Design review of the part built by this model. Coordinates are the model's own, in mm. A direction names the side the tool comes from. Coordinates: 2 decimals unless noted, no trailing zeros. Loops run counter-clockwise (first coordinate to the right, second up) from the corner with the lowest first, then second, coordinate; pieces in that order, holes last. Notation, with made-up numbers: (73.25, 20) -> (101.25, 20) arc R14 ccw to (101.25, 38) -> close; hole circle Ø9 at (-30, 82). An arc over 180 degrees is marked (long way). Answer as a JSON object with one key per item and string values.
```python
from build123d import *

# Parameters (mm, degrees)
SKETCH_1_R          = 32.5
EXTRUDE_1_DEPTH     = 154.5
SKETCH_2_R          = 12.5
EXTRUDE_2_DEPTH     = 6
SKETCH_3_R          = 6
CUT_EXTRUDE_1_DEPTH = 80
SKETCH_4_R          = 8
EXTRUDE_3_DEPTH     = 5
SKETCH_5_R          = 8
EXTRUDE_4_DEPTH     = 2.5
SKETCH_8_R          = 4
SKETCH_7_R          = 6
SKETCH_9_R          = 2.5
CUT_EXTRUDE_2_DEPTH = 31
SKETCH_10_R         = 6
CUT_EXTRUDE_3_DEPTH = 17


with BuildPart() as part:
    # 草图1 → 凸台-拉伸1 (new body)
    with BuildSketch(Plane(origin=(0, 0, 0), x_dir=(1, 0, 0), z_dir=(0, 1, 0))):
        with Locations(Location((0, 0, 0), (0, 0, 270))):
            Circle(SKETCH_1_R)
    extrude(amount=EXTRUDE_1_DEPTH)

    # 草图2 → 凸台-拉伸2 (add)
    with BuildSketch(Plane.XZ):
        with Locations(Location((0, 0, 0), (0, 0, 270))):
            Circle(SKETCH_2_R)
    extrude(amount=EXTRUDE_2_DEPTH)

    # 草图3 → 切除-拉伸1 (cut)
    with BuildSketch(Plane.XZ.offset(6)):
        with Locations(Location((0, 0, 0), (0, 0, 270))):
            Circle(SKETCH_3_R)
    extrude(amount=-CUT_EXTRUDE_1_DEPTH, mode=Mode.SUBTRACT)

    # 草图4 → 凸台-拉伸3 (add, symmetric)
    with BuildSketch(Plane.XY):
        with BuildLine():
            Line((-11, 154.5), (11, 154.5))
            Line((11, 154.5), (11, 164.5))
            ThreePointArc((11, 164.5), (0, 174.786108986), (-11, 164.5))
            Line((-11, 164.5), (-11, 154.5))
        make_face()
        with Locations((0, 163.761335751)):
            Circle(SKETCH_4_R, mode=Mode.SUBTRACT)
    extrude(amount=EXTRUDE_3_DEPTH, both=True)

    # 草图5 → 凸台-拉伸4 (add, symmetric)
    with BuildSketch(Plane.XY):
        with Locations((0, 163.761335751)):
            Circle(SKETCH_5_R)
    extrude(amount=EXTRUDE_4_DEPTH, both=True)

    # 草图8 → 放样1 section 0
    with BuildSketch(Plane.XY.offset(4.5)):
        with Locations((0, 163.761335751)):
            Circle(SKETCH_8_R)
    # 草图7 → 放样1 section 1
    with BuildSketch(Plane.XY.offset(2.5)):
        with Locations((0, 163.761335751)):
            Circle(SKETCH_7_R)
    loft_1 = loft()

    # 镜向1: 放样1 across plane
    add(loft_1.mirror(Plane.XY))

    # 草图9 → 切除-拉伸2 (cut)
    with BuildSketch(Plane.XY.offset(4.5)):
        with Locations(Location((0, 166.761335751, 0), (0, 0, 2.865983983))):
            Circle(SKETCH_9_R)
    extrude(amount=-CUT_EXTRUDE_2_DEPTH, mode=Mode.SUBTRACT)

    # 草图10 → 切除-拉伸3 (cut)
    with BuildSketch(Plane.XY.offset(4.5)):
        with Locations((0, 163.761335751)):
            Circle(SKETCH_10_R)
    extrude(amount=-CUT_EXTRUDE_3_DEPTH, mode=Mode.SUBTRACT)

    # 草图11 → 切除-旋转1 (revolve, cut)
    with BuildSketch(Plane.XY):
        with BuildLine():
            Line((0, 170.261335751), (0, 157.261335751))
            ThreePointArc((0, 157.261335751), (6.5, 163.761335751), (0, 170.261335751))
        make_face()
    revolve(axis=Axis((0, 170.261335751, 0), (0, -1, 0)), mode=Mode.SUBTRACT)


solid = part.part
```
1) Add section B-B, the plane x = 0. Give the boundary of the cut face in (y, z), and give its area (3 significant figures).
Completed:
{"outline": "(-6, -12.5) -> (0, -12.5) -> (0, -32.5) -> (154.5, -32.5) -> (154.5, -5) -> (155.76, -5) -> (155.76, -2.5) -> (157.76, -2.5) arc R6.5 cw to (157.76, 2.5) -> (155.76, 2.5) -> (155.76, 5) -> (154.5, 5) -> (154.5, 32.5) -> (0, 32.5) -> (0, 12.5) -> (-6, 12.5) -> (-6, 6) -> (74, 6) -> (74, -6) -> (-6, -6) -> close; (169.76, -2.5) -> (171.76, -2.5) -> (171.76, -5) -> (174.79, -5) -> (174.79, 5) -> (171.76, 5) -> (171.76, 2.5) -> (169.76, 2.5) arc R6.5 cw to start", "area": "9,290 mm²"}
2) Clearance check with flat-ended pins moving along their axes: pin 1 Ø12 at (x, y) = (17, 156.5) entering from -Z; pin 2 Ø8 at (y, z) = (160.5, 1.5) entering from +X; pin 3 Ø10 at (y, z) = (76, 5) entering from -X; pin 4 Ø15.5 at (x, z) = (0, 0) entering from -Y. State where each tip first meets the part, or that it passes through.
Completed:
{"pin 1": "z = -30.46", "pin 2": "x = 11", "pin 3": "x = -32.5", "pin 4": "y = -6"}
3) For faces 4 (the flat face through (11, 159, 0)), 5 (the flat face through (-7.5, 167, 5)), 6 (the flat face through (1, 170, 2.5)), list the 3-axis set-ups (+Z, -Z, +X, -X, +Y, -Y) from which the entire face can be reached by the end or side of a thin tool; tool diameter is ignored.
Completed:
{"face 4": "+Z, -Z, +X, +Y", "face 5": "+Z, +X, -X, +Y", "face 6": "+Z"}
4) Add section A-A, the plane z = 0. Give the boundary of the cut face in (x, y), and give its area (3 significant figures).
Completed:
{"outline": "(-32.5, 0) -> (-12.5, 0) -> (-12.5, -6) -> (-6, -6) -> (-6, 74) -> (6, 74) -> (6, -6) -> (12.5, -6) -> (12.5, 0) -> (32.5, 0) -> (32.5, 154.5) -> (11, 154.5) -> (11, 164.5) arc R11.02 ccw to (-11, 164.5) -> (-11, 154.5) -> (-32.5, 154.5) -> close; hole circle Ø13 at (0, 163.76)", "area": "9,490 mm²"}
5) The part is to be moulded in two halves that separate along X. For faces 1 (the flat face through (0, 0, 14)), 2 (the cylindrical face through (1.802, 33.44, -5.723)), 3 (the cylindrical face through (3.755, -2.958, -11.923)), say which applies: pulls with the +X half, pulls with the -X half, needs draft (parallel to the pull), parting line crosses it, or undercut.
Completed:
{"face 1": "needs draft", "face 2": "undercut", "face 3": "parting line crosses it"}
6) Wall thickness on probe 1 along Y at (x, z) = (0, -4); probe 2 along Y at (x, z) = (27, 17); probe 3 along Z at (x, y) = (-5.5, 8): over which ranges is each line inside the solid? List them lowest first.
Completed:
{"probe 1": "74 to 155.76, 171.76 to 174.79", "probe 2": "0 to 154.5", "probe 3": "-32.03 to -2.4, 2.4 to 32.03"}
7) Add section C-C, the plane y = 135.5. Give the boundary of the cut face in (x, z).
Completed:
{"outline": "circle Ø65 at (0, 0)"}
8) Add section D-D, the plane y = 54.5. Give the boundary of the cut face in (x, z), and give its area (3 significant figures).
Completed:
{"outline": "circle Ø65 at (0, 0); hole circle Ø12 at (0, 0)", "area": "3,210 mm²"}
